from build123d import *

# Parameters (mm, degrees)
F1_DEPTH = 0.5
F2_R     = 1.5


with BuildPart() as f1:
    # F0 (on Top) → F1 (new body)
    with BuildSketch(Plane.XY):
        with BuildLine():
            Line((-2.4494897428, 2.5), (2.4494897428, 2.5))
            ThreePointArc((2.4494897428, 2.5), (0, 3.5), (-2.4494897428, 2.5))
        make_face()
        with BuildLine():
            ThreePointArc((2.4494897428, -2.5), (3.2267021942, -1.3558735008), (3.5, 0))
            ThreePointArc((3.5, 0), (3.2267021942, 1.3558735008), (2.4494897428, 2.5))
            Line((2.4494897428, 2.5), (-2.4494897428, 2.5))
            ThreePointArc((-2.4494897428, 2.5), (-3.5, 0), (-2.4494897428, -2.5))
            Line((-2.4494897428, -2.5), (2.4494897428, -2.5))
        make_face()
        with BuildLine():
            ThreePointArc((2.4494897428, 2.5), (3.2267021942, 1.3558735008), (3.5, 0))
            ThreePointArc((3.5, 0), (3.2267021942, -1.3558735008), (2.4494897428, -2.5))
            Line((2.4494897428, -2.5), (4, -2.5))
            Line((4, -2.5), (4, 2.5))
            Line((4, 2.5), (2.4494897428, 2.5))
        make_face()
        with BuildLine():
            ThreePointArc((-2.4494897428, -2.5), (0, -3.5), (2.4494897428, -2.5))
            Line((2.4494897428, -2.5), (-2.4494897428, -2.5))
        make_face()
        with BuildLine():
            ThreePointArc((-2.4494897428, -2.5), (-3.5, 0), (-2.4494897428, 2.5))
            Line((-2.4494897428, 2.5), (-4, 2.5))
            Line((-4, 2.5), (-4, -2.5))
            Line((-4, -2.5), (-2.4494897428, -2.5))
        make_face()
    extrude(amount=F1_DEPTH)

    # F2
    f2_edges = [f1.edges().sort_by_distance(p)[0] for p in [
        (-4, -2.5, 0.25),
        (-4, 2.5, 0.25),
        (4, -2.5, 0.25),
        (4, 2.5, 0.25),
    ]]
    fillet(f2_edges, radius=F2_R)


solid = f1.part
Here's how the part is built. I have some questions about the finished solid (model axes, mm). Round coordinates to 2 decimals unless told otherwise and drop trailing zeros. Order: outer loops, then holes, each group sorted by start corner. A loop starts at its lowest first (then second) coordinate and runs counter-clockwise, first axis right, second up. Notation, with made-up numbers: (-19.75, -29) -> (10.25, -29) arc R22 cw to (10.25, -2) -> close; hole circle Ø8 at (48.5, 29). An arc over 180 degrees is marked (long way). Use CSV: the item, a comma, the result in double quotes.
1. I want a section at A-A on z = 0.1. List the corners of the cut face in (x, y) for me, and give its area (3 significant figures).
Recorded:
outline,"(-4, -1) arc R1.5 ccw to (-2.5, -2.5) -> (-2.45, -2.5) arc R3.5 ccw to (2.45, -2.5) -> (2.5, -2.5) arc R1.5 ccw to (4, -1) -> (4, 1) arc R1.5 ccw to (2.5, 2.5) -> (2.45, 2.5) arc R3.5 ccw to (-2.45, 2.5) -> (-2.5, 2.5) arc R1.5 ccw to (-4, 1) -> close"
area,"44.8 mm2"
2. I want a section at B-B on y = -2. List the corners of the cut face in (x, z) for me, and give its area (3 significant figures).
Recorded:
outline,"(-3.62, 0) -> (3.62, 0) -> (3.62, 0.5) -> (-3.62, 0.5) -> close"
area,"3.62 mm2"
3. I want a section at C-C on x = 1.25. List the corners of the cut face in (y, z) for me, and give its area (3 significant figures).
Recorded:
outline,"(-3.27, 0) -> (3.27, 0) -> (3.27, 0.5) -> (-3.27, 0.5) -> close"
area,"3.27 mm2"
4. I'm going to push a flat-ended pin straight in: P1, Ø1, axis at x = -1.5, y = 0, coming from the -Z side. Where does the tip first touch, or does it pass through?
Recorded:
P1,"stops at z = 0"
5. I need wall thicknesses on line 1 along Y through (x, z) = (2.5, 0.2); line 2 along Y through (x, z) = (-0.75, 0.45); line 3 along X through (y, z) = (-2.25, 0.05). Which ranges of each line are inside material? Lowest first, please.
Recorded:
line 1,"y = -2.5 to 2.5"
line 2,"y = -3.42 to 3.42"
line 3,"x = -3.33 to 3.33"
